```python
from build123d import *

# Parameters (mm, degrees)
F0_W      = 52.7558
F0_H      = 45.1358
F1_DEPTH  = 5.08
F2_W      = 3.81
F2_H      = 45.1358
F3_DEPTH  = 5.08
F4_R      = 4.953
F5_DEPTH  = 25.4
F7_DEPTH  = 26.3779
F8_W      = 30.988
F8_H      = 12.7
F9_DEPTH  = 46.7108254453
F10_W     = 30.988
F10_H     = 6.35
F11_DEPTH = 5.08
F12_F1_R  = 1.27
F12_F2_R  = 1.27
F13_W     = 30.988
F13_H     = 7.8715959617
F13_H_2   = 2.2884040383
F14_DEPTH = 25.4


with BuildPart() as f1:
    # F0 (on Top) → F1 (new body)
    with BuildSketch(Plane.XY):
        Rectangle(F0_W, F0_H)
    extrude(amount=F1_DEPTH)

    # F2 (on Top) → F3 (join)
    with BuildSketch(Plane.XY):
        with Locations((24.4729, 0)):
            Rectangle(F2_W, F2_H)
        with Locations((-24.4729, 0)):
            Rectangle(F2_W, F2_H)
    extrude(amount=-F3_DEPTH)

    # F4 (on Top) → F5 (cut)
    with BuildSketch(Plane.XY):
        Circle(F4_R)
    extrude(amount=F5_DEPTH, mode=Mode.SUBTRACT)

    # F6 (on Right) → F7 (join, symmetric)
    with BuildSketch(Plane.YZ):
        Polygon((21.1386244499, 67.4993857748), (-22.5679, 5.08), (-16.3663650891, 5.08), (27.3401593609, 67.4993857748), align=None)
    extrude(amount=F7_DEPTH, both=True)

    # F8 (on face) → F9 (cut, through all)
    with BuildSketch(Plane(origin=(0, -17.5301074531, 12.2747133843), x_dir=(1, 0, 0), z_dir=(0, -0.8191520443, 0.5735764364))):
        with Locations((0, 56.8473525345)):
            Rectangle(F8_W, F8_H)
    extrude(amount=-F9_DEPTH, mode=Mode.SUBTRACT)

    # F10 (on face) → F11 (cut, through all)
    with BuildSketch(Plane(origin=(0, -17.5301074531, 12.2747133843), x_dir=(1, 0, 0), z_dir=(0, -0.8191520443, 0.5735764364))):
        with Locations((0, 9.2223525345)):
            Rectangle(F10_W, F10_H)
    extrude(amount=-F11_DEPTH, mode=Mode.SUBTRACT)

    # F12: fillet of radius 1.27 on 49 edges, made by hand

    # F12_f1
    f12_f1_edges = [f1.edges().sort_by_distance(p)[0] for p in [
        (0, -16.3663650891, 5.08),
        (22.5679, 0, 0),
        (-22.5679, 0, 0),
    ]]
    fillet(f12_f1_edges, radius=F12_F1_R)

    # F12_f2
    f12_f2_edges = [f1.edges().sort_by_distance(p)[0] for p in [
        (26.3779, 4.3205911061, 5.08),
        (26.3779, 22.5679, 0),
        (26.3779, 0, -5.08),
        (26.3779, -22.5679, 0),
        (26.3779, -0.714637775, 36.2896928874),
        (26.3779, 24.2393919054, 67.4993857748),
        (26.3779, 6.1865592384, 37.2889139245),
        (-26.3779, 22.5679, 0),
        (-26.3779, 4.3205911061, 5.08),
        (-26.3779, 6.1865592384, 37.2889139245),
        (-26.3779, 24.2393919054, 67.4993857748),
        (-26.3779, -0.714637775, 36.2896928874),
        (-26.3779, -22.5679, 0),
        (-26.3779, 0, -5.08),
        (0, 21.1386244499, 67.4993857748),
        (0, -22.5679, 5.08),
        (0, 11.4339840588, 53.6397229441),
        (-15.494, 15.0761944297, 58.8413384253),
        (15.494, 15.0761944297, 58.8413384253),
        (0, 18.7184048005, 64.0429539066),
        (0, -14.061488537, 17.2284145755),
        (15.494, -12.2403833515, 19.8292223161),
        (0, -10.4192781661, 22.4300300567),
        (-15.494, -12.2403833515, 19.8292223161),
        (0, 27.3401593609, 67.4993857748),
        (-15.494, -8.0790909666, 16.9154540194),
        (0, -6.2579857811, 19.51626176),
        (15.494, -8.0790909666, 16.9154540194),
        (0, -9.900196152, 14.3146462788),
        (0, 15.5952764438, 50.7259546475),
        (15.494, 19.2374868147, 55.9275701287),
        (-15.494, 19.2374868147, 55.9275701287),
        (0, 22.8796971855, 61.1291856099),
        (0, 22.5679, 5.08),
        (-4.953, 0, 5.08),
        (-24.4729, 22.5679, -5.08),
        (-22.5679, 22.5679, -3.175),
        (0, 22.5679, 0),
        (22.5679, 22.5679, -3.175),
        (24.4729, 22.5679, -5.08),
        (-22.5679, -22.5679, -3.175),
        (-22.5679, 0, -5.08),
        (24.4729, -22.5679, -5.08),
        (22.5679, 0, -5.08),
        (-24.4729, -22.5679, -5.08),
        (0, -22.5679, 0),
        (-22.1959256121, -22.5679, -0.3719743879),
        (22.1959256121, -22.5679, -0.3719743879),
        (22.1959256121, 22.5679, -0.3719743879),
        (-22.1959256121, 22.5679, -0.3719743879),
        (-26.3779, -15.053221546, 5.7635792612),
        (26.3779, -15.053221546, 5.7635792612),
    ]]
    fillet(f12_f2_edges, radius=F12_F2_R)

    # F13 (on face) → F14 (cut)
    with BuildSketch(Plane(origin=(0, -17.5301074531, 12.2747133843), x_dir=(1, 0, 0), z_dir=(0, -0.8191520443, 0.5735764364))):
        with Locations((0, 70.6915545537)):
            Rectangle(F13_W, F13_H)
        with Locations((0, 65.6115545537)):
            Rectangle(F13_W, F13_H_2)
        Polygon((-15.494, 63.4007958817), (-15.494, 56.8473525345), (15.494, 56.8473525345), (15.494, 64.4673525345), (-15.494, 64.4673525345), align=None)
    extrude(amount=-F14_DEPTH, mode=Mode.SUBTRACT)


solid = f1.part
```
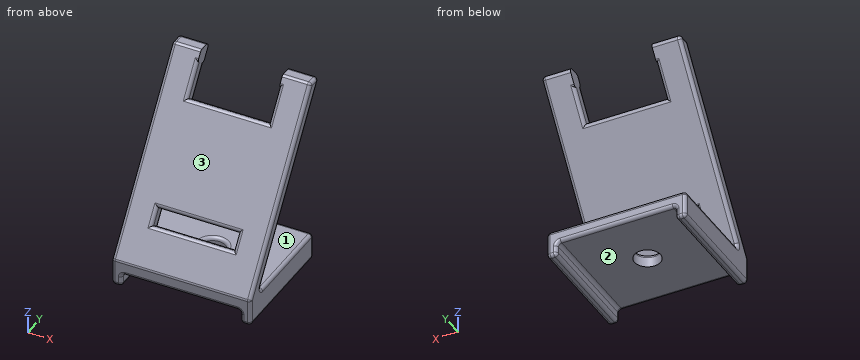
Design review of the part built by this model. Coordinates are the model's own, in mm. Face numbers are marked on the shaded views. A direction names the side the tool comes from. Coordinates: 2 decimals unless noted, no trailing zeros. Order: outer loops, then holes, each group sorted by start corner. A loop starts at its lowest first (then second) coordinate and runs counter-clockwise, first axis right, second up. Notation, with made-up numbers: (-9, 39.25) -> (10, 39.25) arc R27 cw to (10, 64.25) -> close; hole circle Ø7 at (26.5, 27.25). An arc over 180 degrees is marked (long way). One line per item, written item: value. Start each with the question number.
Q1. For probe 1 along Y at (x, z) = (0, 1.4); probe 2 along X at (y, z) = (0, 2.4); probe 3 along Z at (x, y) = (21, -15), list the stretches that pass through material, from the lowest coordinate up.
Q2. Tool access review of the marked faces 1, 2 and 3: name each direction out of +Z, -Z, +X, -X, +Y, -Y from which nothing blocks a thin tool from reaching the whole face with its end or side.
Q3. Take a section at A-A, the plane x = 0. State the section outline as (y, z) points, then the cut area to 3 significant figures.
Q4. Take a section at B-B, the plane x = -10. State the section outline as (y, z) points.
Q5. Insertion check: pin 1 Ø1.5 at (x, z) = (5, 14.5) entering from -Y; pin 2 Ø4 at (x, y) = (4.5, 18.5) entering from +Z; pin 3 Ø6 at (x, y) = (0, 0) entering from +Z. Each pin has a flat end and moves straight along its axis. Give the tip position at first contact, or say it passes through.
Q6. Take a section at C-C, the plane y = 2. Give the number of separate pieces and of enclosed holes in the cut face, then the cut area to 3 significant figures.
Values follow:
1. probe 1: y = -22.57 to -4.95, 4.95 to 22.57
1. probe 2: x = -26.38 to -4.95, 4.95 to 26.38
1. probe 3: z = 0 to 5.67, 7.03 to 15.89
2. face 1: +X, -X, +Y
2. face 2: -Z, +Y, -Y
2. face 3: +Z, +X, -X, -Y
3. outline: (-22.57, 1.27) arc R1.27 ccw to (-21.3, 0) -> (-4.95, 0) -> (-4.95, 3.81) arc R1.27 ccw to (-6.22, 5.08) -> (-13.93, 5.08) arc R1.27 cw to (-14.97, 7.08) -> (-10.63, 13.27) arc R1.27 ccw to (-10.94, 15.04) -> (-13.02, 16.5) arc R1.27 ccw to (-14.79, 16.19) -> (-22.34, 5.41) arc R1.27 ccw to (-22.57, 4.68) -> close; (-9.69, 23.47) arc R1.27 ccw to (-9.38, 21.7) -> (-7.3, 20.24) arc R1.27 ccw to (-5.53, 20.56) -> (14.87, 49.69) arc R1.27 ccw to (14.55, 51.45) -> (12.47, 52.91) arc R1.27 ccw to (10.71, 52.6) -> close; (4.95, 0) -> (21.3, 0) arc R1.27 ccw to (22.57, 1.27) -> (22.57, 3.81) arc R1.27 ccw to (21.3, 5.08) -> (6.22, 5.08) arc R1.27 ccw to (4.95, 3.81) -> close
3. area: 436 mm2
4. outline: (-22.57, 1.27) arc R1.27 ccw to (-21.3, 0) -> (21.3, 0) arc R1.27 ccw to (22.57, 1.27) -> (22.57, 3.81) arc R1.27 ccw to (21.3, 5.08) -> (-13.93, 5.08) arc R1.27 cw to (-14.97, 7.08) -> (-10.63, 13.27) arc R1.27 ccw to (-10.94, 15.04) -> (-13.02, 16.5) arc R1.27 ccw to (-14.79, 16.19) -> (-22.34, 5.41) arc R1.27 ccw to (-22.57, 4.68) -> close; (-9.69, 23.47) arc R1.27 ccw to (-9.38, 21.7) -> (-7.3, 20.24) arc R1.27 ccw to (-5.53, 20.56) -> (14.87, 49.69) arc R1.27 ccw to (14.55, 51.45) -> (12.47, 52.91) arc R1.27 ccw to (10.71, 52.6) -> close
5. pin 1: stops at y = -16.5
5. pin 2: stops at z = 5.08
5. pin 3: stops at z = 41.59
6. separate pieces: 3
6. enclosed holes: 0
6. area: 723 mm2
